```python
from build123d import *

# Parameters (mm, degrees)
SKETCH1_R                = 47.25
BOSS_EXTRUDE1_DEPTH      = 6
SKETCH2_R                = 1.1
CUT_EXTRUDE1_DEPTH       = 20
M5_CLEARANCE_HOLE1_D     = 5.3
M5_CLEARANCE_HOLE1_DEPTH = 15
M5_CLEARANCE_HOLE1_TIP   = 1.59228064


with BuildPart() as part:
    # Sketch1 → Boss-Extrude1 (new body)
    with BuildSketch(Plane(origin=(0, 0, 0), x_dir=(0, 0, -1), z_dir=(1, 0, 0))):
        Circle(SKETCH1_R)
    extrude(amount=BOSS_EXTRUDE1_DEPTH)

    # Sketch2 → Cut-Extrude1 (cut)
    with BuildSketch(Plane(origin=(6, 0, 0), x_dir=(0, 0, -1), z_dir=(1, 0, 0))):
        with BuildLine():
            Line((12, -2.85), (-12, -2.85))
            ThreePointArc((-12, -2.85), (-12.812754403, -3.224796478), (-13, -4.1))
            Line((-13, -4.1), (-13, -10.85))
            ThreePointArc((-13, -10.85), (-12.707106781, -11.557106781), (-12, -11.85))
            Line((-12, -11.85), (12, -11.85))
            ThreePointArc((12, -11.85), (12.707106781, -11.557106781), (13, -10.85))
            Line((13, -10.85), (13, -3.85))
            ThreePointArc((13, -3.85), (12.707106781, -3.142893219), (12, -2.85))
        make_face()
        with BuildLine():
            ThreePointArc((-12, -11.85), (-12.707106781, -11.557106781), (-13, -10.85))
            Line((-13, -10.85), (-13, -11.85))
            ThreePointArc((-13, -11.85), (-12.707106781, -12.557106781), (-12, -12.85))
            Line((-12, -12.85), (12, -12.85))
            ThreePointArc((12, -12.85), (12.707106781, -12.557106781), (13, -11.85))
            Line((13, -11.85), (13, -10.85))
            ThreePointArc((13, -10.85), (12.707106781, -11.557106781), (12, -11.85))
            Line((12, -11.85), (-12, -11.85))
        make_face()
        with Locations((-10.5, 0.25)):
            Circle(SKETCH2_R)
        with Locations((10.5, 0.25)):
            Circle(SKETCH2_R)
        with Locations((10.5, 12.75)):
            Circle(SKETCH2_R)
        with Locations((-10.5, 12.75)):
            Circle(SKETCH2_R)
    extrude(amount=-CUT_EXTRUDE1_DEPTH, mode=Mode.SUBTRACT)

    # M5 Clearance Hole1
    with Locations(Plane(origin=(6, 0, 0), x_dir=(0, 0, -1), z_dir=(1, 0, 0))):
        with Locations((-32, 0), (0, 32), (32, 0), (0, -32)):
            Hole(M5_CLEARANCE_HOLE1_D / 2, depth=M5_CLEARANCE_HOLE1_DEPTH)
            with Locations((0, 0, -(M5_CLEARANCE_HOLE1_DEPTH + M5_CLEARANCE_HOLE1_TIP / 2))):  # 118° drill point
                Cone(0, M5_CLEARANCE_HOLE1_D / 2, M5_CLEARANCE_HOLE1_TIP, mode=Mode.SUBTRACT)


solid = part.part
```
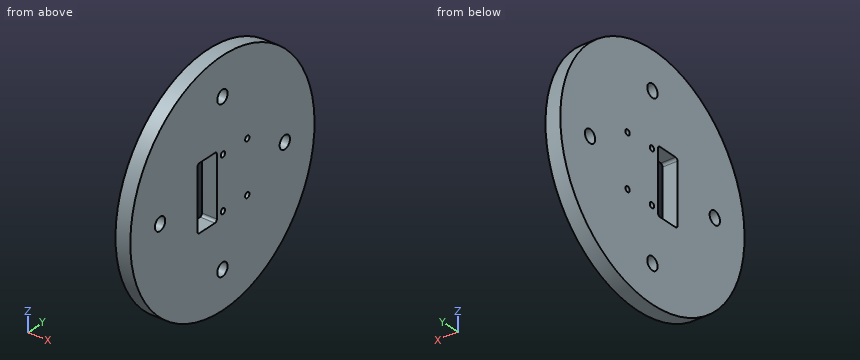
Read the model definition and answer for the solid it produces. Units are mm, in the model's axes. Round coordinates to 2 decimals unless told otherwise and drop trailing zeros. Write each loop counter-clockwise with the first axis right and the second up, starting at its lowest first coordinate (ties: lowest second). Pieces come first, ordered by that corner, then holes. Notation, with made-up numbers: (71, 42.5) - (96, 42.5) arc R9 ccw to (96, 46.5) - close; hole circle Ø9 at (-33, 36.5). An arc over 180 degrees is marked (long way). One line per item, written item: value.
Q1. Find section A-A (x = 1.8). Count the separate pieces of the cut face and the enclosed holes in it, and give its area (3 significant figures).
The answers:
separate pieces: 1
enclosed holes: 9
area: 6,650 mm2
Q2. Straight lines are drawn through the part: line 1 (Y direction, x = 1.6, z = 0); line 2 (Y direction, x = 1.45, z = -10.5); line 3 (Z direction, x = 5.5, y = 12.5). For each, find the intervals that lie inside material, in ascending order. Write a range as from..to.
The answers:
line 1: y = -47.25..-34.65, -29.35..-12.85, -2.85..29.35, 34.65..47.25
line 2: y = -46.07..-12.85, -2.85..-0.85, 1.35..11.65, 13.85..46.07
line 3: z = -45.57..-11.57, -9.43..9.43, 11.57..45.57
Q3. Find section B-B (z = 10.5). Determine the outline of the cut face in (x, y), and give its area (3 significant figures).
The answers:
outline: (0, -46.07) - (6, -46.07) - (6, -12.85) - (0, -12.85) - close; (0, -2.85) - (6, -2.85) - (6, -0.85) - (0, -0.85) - close; (0, 1.35) - (6, 1.35) - (6, 11.65) - (0, 11.65) - close; (0, 13.85) - (6, 13.85) - (6, 46.07) - (0, 46.07) - close
area: 466 mm2
Q4. Each of these flat-tipped pins is pushed along its axis until it touches: P1, Ø3, axis at x = 2.5, z = -4.5, coming from the +Y side; P2, Ø4, axis at y = 0, z = 32, coming from the +X side; P3, Ø8.5, axis at y = 32, z = 0, coming from the +X side; P4, Ø2, axis at x = 4.5, z = -20, coming from the -Y side. Where does it stop, or does it pass through?
The answers:
P1: stops at y = 47.15
P2: passes through
P3: stops at x = 6
P4: stops at y = -43.26
Q5. Find section C-C (y = -32). Determine the outline of the cut face in (x, z), and give its area (3 significant figures).
The answers:
outline: (0, -34.76) - (6, -34.76) - (6, -2.65) - (0, -2.65) - close; (0, 2.65) - (6, 2.65) - (6, 34.76) - (0, 34.76) - close
area: 385 mm2
